```python
from build123d import *

# Parameters (mm, degrees)
SKETCH_1_W               = 500
SKETCH_1_H               = 110
SKETCH_1_R               = 16.844258013
SKETCH_1_R_2             = 10
EXTRUDE_1_DEPTH          = 20
CUT_EXTRUDE_1_DEPTH      = 274.861278753
CUT_EXTRUDE_1_DEPTH_BACK = 274.861278753


with BuildPart() as part:
    # 草图1 → 凸台-拉伸1 (new body)
    with BuildSketch(Plane.XY):
        with Locations((0, 55)):
            Rectangle(SKETCH_1_W, SKETCH_1_H)
        with Locations((175.900033463, 52.997126546)):
            Circle(SKETCH_1_R, mode=Mode.SUBTRACT)
        with Locations((-175.9468126, 13.777754179)):
            Circle(SKETCH_1_R_2, mode=Mode.SUBTRACT)
        with Locations((-201.422811837, 59.841384559)):
            Circle(SKETCH_1_R_2, mode=Mode.SUBTRACT)
    extrude(amount=EXTRUDE_1_DEPTH)

    # 草图2 → 切除-拉伸1 (cut, two sides: drawn at the far end of the back side and taken through both)
    with BuildSketch(Plane.XY.offset(20).offset(-CUT_EXTRUDE_1_DEPTH_BACK)):
        Polygon((1297.820746048, 138.80913238), (250, 138.80913238), (210, 138.80913238), (210, -127.893820907), (210, -1175.714566955), (1824.507064902, -2511.783502593), (2912.32781095, -1197.259803259), align=None)
    extrude(amount=CUT_EXTRUDE_1_DEPTH + CUT_EXTRUDE_1_DEPTH_BACK, mode=Mode.SUBTRACT)


solid = part.part
```
Input: part model. Units: mm. Frame: model coordinates. Coordinates: 2 decimals unless noted, no trailing zeros. Write each loop counter-clockwise with the first axis right and the second up, starting at its lowest first coordinate (ties: lowest second). Pieces come first, ordered by that corner, then holes. Notation, with made-up numbers: M -10,26.5 L 35,26.5 A33 ccw 35,54.5 Z; hole C -24,70 d5. An arc over 180 degrees is marked long. Use one line per item in the form item = value.
Q1. Section C-C (y = 46). Return loops of the section in (x, z).
Answer below:
outline = M -250,0 L 160.58,0 L 160.58,20 L -250,20 Z; M 191.22,0 L 210,0 L 210,20 L 191.22,20 Z
Q2. Material intervals for probe 1 along X at (y, z) = (55, 12.5); probe 2 along X at (y, z) = (40.5, 10); probe 3 along Y at (x, z) = (189, 17), sorted ascending. Write a range as from..to.
Answer below:
probe_1 = -250..-210.17, -192.67..159.18, 192.62..210
probe_2 = -250..164.61, 187.19..210
probe_3 = 0..42.41, 63.59..110
Q3. Section B-B (z = 16). Return loops of the section in (x, y).
Answer below:
outline = M -250,0 L 210,0 L 210,110 L -250,110 Z; hole C -201.42,59.84 d20; hole C -175.95,13.78 d20; hole C 175.9,53 d33.69
Q4. First-contact query: pin 1 (18 mm diameter, centred on x = -201.42, y = 59.84, fed in from -Z); pin 2 (10 mm diameter, centred on x = -175, z = 3, fed in from -Y). Flat tips, straight axial feed; report the tip coordinate or a pass-through.
Answer below:
pin_1 = through
pin_2 = 0
Q5. Section A-A (y = 18). Return loops of the section in (x, z).
Answer below:
outline = M -250,0 L -185.01,0 L -185.01,20 L -250,20 Z; M -166.88,0 L 210,0 L 210,20 L -166.88,20 Z
Q6. Draft query along X for faces 1 (the face through (-196.81, 50.97, 9.86)), 2 (the face through (-250, 54, 10)), 3 (the face through (-23, 56, 20)). Return one class per face: released by +X, released by -X, zero draft, split by the parting line, or undercut.
Answer below:
face_1 = undercut
face_2 = released by -X
face_3 = zero draft
